```python
from build123d import *

# Parameters (mm, degrees)
EXTRUDE_1_DEPTH        = 195
SKETCH_2_R             = 3
SKETCH_2_R_2           = 1.75
CUT_EXTRUDE_1_DEPTH    = 4.5
SKETCH_2_2_R           = 1.75
CUT_EXTRUDE_2_DEPTH    = 9
PATTERN_LINEAR_1_COUNT = 12
PATTERN_LINEAR_1_PITCH = 25


with BuildPart() as part:
    # Эскиз1 → Бобышка-Вытянуть1 (new body)
    with BuildSketch(Plane.XY):
        with BuildLine():
            Line((-6, 3.7), (-5.7, 4))
            Line((-5.7, 4), (5.7, 4))
            Line((5.7, 4), (6, 3.7))
            Line((6, 3.7), (6, 2.449776022))
            ThreePointArc((6, 2.449776022), (5.561887715, 2.168810579), (5.297911886, 1.720256551))
            Line((5.297911886, 1.720256551), (4.687472904, 1.720256551))
            Line((4.687472904, 1.720256551), (4.687472904, 1.082255421))
            Line((4.687472904, 1.082255421), (5.292171789, 1.082255421))
            ThreePointArc((5.292171789, 1.082255421), (5.554928022, 0.621665058), (6, 0.333402583))
            Line((6, 0.333402583), (6, -3.7))
            Line((6, -3.7), (5.7, -4))
            Line((5.7, -4), (-5.7, -4))
            Line((-5.7, -4), (-6, -3.7))
            Line((-6, -3.7), (-6, 0.333402583))
            ThreePointArc((-6, 0.333402583), (-5.554928022, 0.621665058), (-5.292171789, 1.082255421))
            Line((-5.292171789, 1.082255421), (-4.687472904, 1.082255421))
            Line((-4.687472904, 1.082255421), (-4.687472904, 1.720256551))
            Line((-4.687472904, 1.720256551), (-5.297911886, 1.720256551))
            ThreePointArc((-5.297911886, 1.720256551), (-5.561887715, 2.168810579), (-6, 2.449776022))
            Line((-6, 2.449776022), (-6, 3.7))
        make_face()
    extrude(amount=EXTRUDE_1_DEPTH)

    # Эскиз2 → Вырез-Вытянуть1 (cut)
    with BuildSketch(Plane(origin=(0, 4, 0), x_dir=(1, 0, 0), z_dir=(0, 1, 0))):
        with Locations((0.188190244, -10)):
            Circle(SKETCH_2_R)
        with Locations((0.188190244, -10)):
            Circle(SKETCH_2_R_2, mode=Mode.SUBTRACT)
    cut_extrude_1 = extrude(amount=-CUT_EXTRUDE_1_DEPTH, mode=Mode.SUBTRACT)

    # Эскиз2<2> → Вырез-Вытянуть2 (cut, through all)
    with BuildSketch(Plane(origin=(0, 4, 0), x_dir=(1, 0, 0), z_dir=(0, 1, 0))):
        with Locations((0.188190244, -10)):
            Circle(SKETCH_2_2_R)
    cut_extrude_2 = extrude(amount=-CUT_EXTRUDE_2_DEPTH, mode=Mode.SUBTRACT)

    # Линейный массив1: Вырез-Вытянуть1, Вырез-Вытянуть2 ×12
    with Locations(*[(0, 0, i * PATTERN_LINEAR_1_PITCH) for i in range(1, PATTERN_LINEAR_1_COUNT)]):
        add(cut_extrude_1, mode=Mode.SUBTRACT)
        add(cut_extrude_2, mode=Mode.SUBTRACT)


solid = part.part
```
Can you work these out from the model? Positions are in its coordinate system, mm. A direction names the side the tool comes from. Give positions to 0.01 mm unless a question says otherwise; leave off trailing zeros. Loops run counter-clockwise (first coordinate to the right, second up) from the corner with the lowest first, then second, coordinate; pieces in that order, holes last. Notation, with made-up numbers: M 78.5,-6.5 L 128.5,-6.5 A30 cw 128.5,28.5 Z; hole C 5.5,-31 d1. An arc over 180 degrees is marked long. One line per item, written item: value.
(1) Suppose I cut it at A-A on z = 135. List the corners of the cut face in (x, y) for me, plus the area to 3 significant figures.
Returned:
outline: M -6,-3.7 L -5.7,-4 L -1.56,-4 L -1.56,-0.5 L -2.81,-0.5 L -2.81,4 L -5.7,4 L -6,3.7 L -6,2.45 A1.12 cw -5.3,1.72 L -4.69,1.72 L -4.69,1.08 L -5.29,1.08 A1.12 cw -6,0.33 Z; M 1.94,-4 L 5.7,-4 L 6,-3.7 L 6,0.33 A1.12 cw 5.29,1.08 L 4.69,1.08 L 4.69,1.72 L 5.3,1.72 A1.12 cw 6,2.45 L 6,3.7 L 5.7,4 L 3.19,4 L 3.19,-0.5 L 1.94,-0.5 Z
area: 53.5 mm^2
(2) Will these pins go through, and if not, where does the flat tip stop? pin 1 (3 mm diameter, centred on x = 0.19, z = 160, fed in from -Y); pin 2 (1.8 mm diameter, centred on x = 0.5, z = 184, fed in from +Y).
Returned:
pin 1: through
pin 2: y = -0.5
(3) I need wall thicknesses on line 1 (Y direction, x = -5.25, z = 92.5); line 2 (X direction, y = 1.25, z = 65); line 3 (X direction, y = 1.25, z = 135.5). Which ranges of each line are inside material? Lowest first, please.
Returned:
line 1: -4 to 1.08, 1.72 to 4
line 2: -4.69 to 4.69
line 3: -4.69 to -2.77, 3.15 to 4.69
(4) We'd pull the mould along Z, two halves only. Please class faces 3 (the face through (6, -2, 96)), 4 (the face through (0, 0, 195)), 5 (the face through (0, -0.5, 37)): released by +Z, released by -Z, zero draft, split by the parting line, or undercut.
Returned:
face 3: zero draft
face 4: released by +Z
face 5: undercut
(5) Suppose I cut it at B-B on z = 23.5. List the corners of the cut face in (x, y) for me, plus the area to 3 significant figures.
Returned:
outline: M -6,-3.7 L -5.7,-4 L 5.7,-4 L 6,-3.7 L 6,0.33 A1.12 cw 5.29,1.08 L 4.69,1.08 L 4.69,1.72 L 5.3,1.72 A1.12 cw 6,2.45 L 6,3.7 L 5.7,4 L -5.7,4 L -6,3.7 L -6,2.45 A1.12 cw -5.3,1.72 L -4.69,1.72 L -4.69,1.08 L -5.29,1.08 A1.12 cw -6,0.33 Z
area: 92.8 mm^2
(6) Which directions (+Z, -Z, +X, -X, +Y, -Y) give clear straight access to the entire face, cutting with the end or side of a thin tool? Please do faces 1 (the face through (0, -4, 96)), 2 (the face through (2.1, -0.5, 185)).
Returned:
face 1: +Z, -Z, +X, -X, -Y
face 2: +Y
